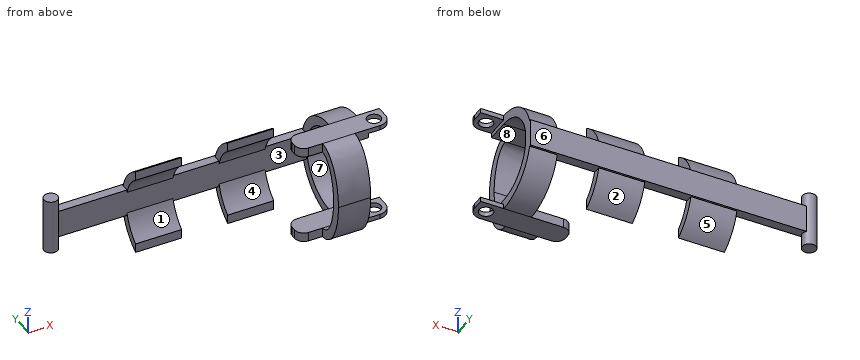
```python
from build123d import *

# Parameters (mm, degrees)
SKETCH1_W                = 2
SKETCH1_H                = 5
BOSS_EXTRUDE1_DEPTH      = 15
BOSS_EXTRUDE1_2_DEPTH    = 15
SKETCH2_W                = 1
SKETCH2_H                = 5
BOSS_EXTRUDE2_DEPTH      = 5
CUT_EXTRUDE1_DEPTH       = 30.107559156
CUT_EXTRUDE1_DEPTH_BACK  = 30.107559156
SKETCH3_R                = 1.5
SWEEP1_START             = 9
SWEEP1_DEPTH             = 6
BOSS_EXTRUDE3_DEPTH      = 12
CUT_EXTRUDE2_DEPTH       = 5
FILLET1_R                = 2
BOSS_EXTRUDE6_START      = -6
SKETCH7_W                = 6
SKETCH7_H                = 2
BOSS_EXTRUDE6_DEPTH      = 61
BOSS_EXTRUDE7_DEPTH      = 3
BOSS_EXTRUDE7_DEPTH_BACK = 9
SKETCH8_R                = 1.5
FILLET2_R                = 2.5
BOSS_EXTRUDE10_DEPTH     = 10
LPATTERN1_COUNT          = 2
LPATTERN1_PITCH          = 20


# Read off the part's stored shape, not the designer's step: Sweep1
with BuildPart() as part:
    # Sketch1 → Boss-Extrude1 (new body)
    with BuildSketch(Plane(origin=(0, 0, 0), x_dir=(0, 0, -1), z_dir=(1, 0, 0))):
        with Locations((-10, 0)):
            Rectangle(SKETCH1_W, SKETCH1_H)
    extrude(amount=BOSS_EXTRUDE1_DEPTH)



with BuildPart() as body_2:
    # Sketch1 → Boss-Extrude1 2 (new body)
    with BuildSketch(Plane(origin=(0, 0, 0), x_dir=(0, 0, -1), z_dir=(1, 0, 0))):
        with Locations((10, 0)):
            Rectangle(SKETCH1_W, SKETCH1_H)
    extrude(amount=BOSS_EXTRUDE1_2_DEPTH)


with BuildPart() as part_1:
    add(part.part)

    add(body_2.part)  # Boss-Extrude2 merges body 2
    # Sketch2 → Boss-Extrude2 (add)
    with BuildSketch(Plane(origin=(15, 0, 0), x_dir=(0, 0, -1), z_dir=(1, 0, 0))):
        with Locations((10.5, 0)):
            Rectangle(SKETCH2_W, SKETCH2_H)
        with Locations((-10.5, 0)):
            Rectangle(SKETCH2_W, SKETCH2_H)
    extrude(amount=BOSS_EXTRUDE2_DEPTH)

    # Sketch3 → Cut-Extrude1 (cut, two sides: drawn at the far end of the back side and taken through both)
    with BuildSketch(Plane.XY.offset(-10).offset(-CUT_EXTRUDE1_DEPTH_BACK)):
        with Locations((17.5, 0)):
            Circle(SKETCH3_R)
    extrude(amount=CUT_EXTRUDE1_DEPTH + CUT_EXTRUDE1_DEPTH_BACK, mode=Mode.SUBTRACT)

    # Sweep1 outline → Sweep1 (add)
    with BuildSketch(Plane.YZ.offset(SWEEP1_START)):
        with BuildLine():
            ThreePointArc((2.5, -11), (13.5, 0), (2.5, 11))
            Line((2.5, 11), (2.5, 9))
            ThreePointArc((2.5, 9), (11.5, 0), (2.5, -9))
            Line((2.5, -9), (2.5, -11))
        make_face()
    extrude(amount=SWEEP1_DEPTH)

    # Sketch5 → Boss-Extrude3 (add)
    with BuildSketch(Plane(origin=(0, 0, 0), x_dir=(0, 0, -1), z_dir=(1, 0, 0))):
        with BuildLine():
            Line((-9, -2.5), (-11, -2.5))
            add(Edge.make_bspline(
                [(-11, -2.5), (-11, -8.980170496), (0, -8.980170496)],
                knots=[3.141592654, 3.141592654, 3.141592654, 4.71238898, 4.71238898, 4.71238898], degree=2, weights=[1, 0.707106781, 1]))
            Line((0, -8.980170496), (0, -7.009343108))
            add(Edge.make_bspline(
                [(-9, -2.5), (-9, -7.009343108), (0, -7.009343108)],
                knots=[3.141592654, 3.141592654, 3.141592654, 4.71238898, 4.71238898, 4.71238898], degree=2, weights=[1, 0.707106781, 1]))
        make_face()
    boss_extrude3 = extrude(amount=BOSS_EXTRUDE3_DEPTH)

    # Sketch6 → Cut-Extrude2 (cut)
    with BuildSketch(Plane.ZY):
        with BuildLine():
            Line((11, -2.5), (9, -2.5))
            add(Edge.make_bspline(
                [(0, -7.009343108), (9, -7.009343108), (9, -2.5)],
                knots=[4.71238898, 4.71238898, 4.71238898, 6.283185307, 6.283185307, 6.283185307], degree=2, weights=[1, 0.707106781, 1]))
            Line((0, -7.009343108), (0, -8.980170496))
            add(Edge.make_bspline(
                [(0, -8.980170496), (11, -8.980170496), (11, -2.5)],
                knots=[4.71238898, 4.71238898, 4.71238898, 6.283185307, 6.283185307, 6.283185307], degree=2, weights=[1, 0.707106781, 1]))
        make_face()
    cut_extrude2 = extrude(amount=-CUT_EXTRUDE2_DEPTH, mode=Mode.SUBTRACT)

    # Mirror2: Boss-Extrude3, Cut-Extrude2 across plane
    add(boss_extrude3.mirror(Plane(origin=(12, -8.980170496, 0), x_dir=(1, 0, 0), z_dir=(0, 0, 1))))
    add(cut_extrude2.mirror(Plane(origin=(12, -8.980170496, 0), x_dir=(1, 0, 0), z_dir=(0, 0, 1))), mode=Mode.SUBTRACT)

    # Fillet1
    fillet1_edges = [part_1.edges().sort_by_distance(p)[0] for p in [
        (0, -2.5, -10),
        (0, 2.5, -10),
        (0, 2.5, 10),
        (0, -2.5, 10),
    ]]
    fillet(fillet1_edges, radius=FILLET1_R)

    # Sketch7 → Boss-Extrude6 (add)
    with BuildSketch(Plane.ZY.offset(-9).offset(BOSS_EXTRUDE6_START)):
        with Locations((0, 12.5)):
            Rectangle(SKETCH7_W, SKETCH7_H)
    extrude(amount=BOSS_EXTRUDE6_DEPTH)

    # Sketch8 → Boss-Extrude7 (add, two sides: drawn at the far end of the back side and taken through both)
    with BuildSketch(Plane.XY.offset(3).offset(-BOSS_EXTRUDE7_DEPTH_BACK)):
        with Locations((-46, 12.5)):
            Circle(SKETCH8_R)
    extrude(amount=BOSS_EXTRUDE7_DEPTH + BOSS_EXTRUDE7_DEPTH_BACK)

    # Fillet2
    fillet2_edges = [part_1.edges().sort_by_distance(p)[0] for p in [
        (20, -2.5, -10.5),
        (20, -2.5, 10.5),
    ]]
    fillet(fillet2_edges, radius=FILLET2_R)

    # 3DSketch3 → Boss-Extrude10 (add)
    with BuildSketch(Plane(origin=(-10, 7.995255445, 9.529017137), x_dir=(0, 0, -1), z_dir=(1, 0, 0))):
        with BuildLine():
            Line((0, 0), (2, 0))
            ThreePointArc((2, 0), (9.529017137, 3.825899604), (17.058034273, 0))
            Line((17.058034273, 0), (19.058034273, 0))
            ThreePointArc((19.058034273, 0), (15.031388903, 4.029654263), (9.529017137, 5.504744555))
            ThreePointArc((9.529017137, 5.504744555), (4.026645371, 4.029654263), (0, 0))
        make_face()
    boss_extrude10 = extrude(amount=BOSS_EXTRUDE10_DEPTH)

    # LPattern1: Boss-Extrude10 ×2
    with Locations(*[(-i * LPATTERN1_PITCH, 0, 0) for i in range(1, LPATTERN1_COUNT)]):
        add(boss_extrude10)


solid = part_1.part
```
Here's how the part is built. I have some questions about the finished solid (model axes, mm). Face numbers are marked on the shaded views. A direction names the side the tool comes from. Round coordinates to 2 decimals unless told otherwise and drop trailing zeros. Order: outer loops, then holes, each group sorted by start corner. A loop starts at its lowest first (then second) coordinate and runs counter-clockwise, first axis right, second up. Notation, with made-up numbers: M -37.5,70.25 L -26.5,70.25 A24 ccw -26.5,95.25 Z; hole C 87,55.5 d6. An arc over 180 degrees is marked long. Use CSV: the item, a comma, the result in double quotes.
1) I want a section at A-A (x = 4). List the corners of the cut face in (y, z) for me.
Taken from the geometry:
outline,"M -2.5,-11 L 2.5,-11 L 2.5,-9 L -2.5,-9 Z; M -2.5,9 L 2.5,9 L 2.5,11 L -2.5,11 Z; M 11.5,-3 L 13.5,-3 L 13.5,3 L 11.5,3 Z"
2) I need wall thicknesses on line 1 along Y through (x, z) = (17.5, 10.4); line 2 along X through (y, z) = (0, 10.75); line 3 along Y through (x, z) = (11, 0). Which ranges of each line are inside material? Lowest first, please. Write a range as [from, to].
Taken from the geometry:
line 1,"[-2.5, -1.5], [1.5, 2.5]"
line 2,"[0, 16], [19, 20]"
line 3,"[-8.98, -7.01], [11.5, 13.5]"
3) I'm going to push flat-ended pins straight in: P1, Ø3, axis at x = -8, z = 6.5, coming from the +Y side; P2, Ø2.5, axis at x = -46.5, y = 12.5, coming from the +Z side; P3, Ø2, axis at x = -16, y = 12, coming from the +Z side. Where does each tip first touch, or does it pass through?
Taken from the geometry:
P1,"y = 12.3"
P2,"z = 6"
P3,"z = 3"
4) If we mould it in two halves opening along X, with no side actions, what happens to the marked faces 1, 2 and 3? For each: pulls with the +X half, pulls with the -X half, needs draft (parallel to the pull), parting line crosses it, or undercut.
Taken from the geometry:
face 1,"undercut"
face 2,"needs draft"
face 3,"undercut"
5) On a 3-axis mill with a long thin cutter (end or side, diameter ignored), from which of +Z, -Z, +X, -X, +Y, -Y can I reach the whole of each face in a straight line? I mean the marked faces 4, 5, 6, 7 and 8. Say none if no direction works.
Taken from the geometry:
face 4,"-Y"
face 5,"-Z, +X, +Y"
face 6,"+Z, -Z, +X, +Y"
face 7,"+X"
face 8,"+X, -X"
6) I want a section at D-D (x = -46). List the corners of the cut face in (y, z) for me, then the cut area to 3 significant figures.
Taken from the geometry:
outline,"M 11,-6 L 14,-6 L 14,6 L 11,6 Z"
area,"36.0 mm^2"
7) I want a section at B-B (y = 3.25). List the corners of the cut face in (x, z) for me.
Taken from the geometry:
outline,"M 9,-10.97 L 15,-10.97 L 15,-8.97 L 9,-8.97 Z; M 9,8.97 L 15,8.97 L 15,10.97 L 9,10.97 Z"
8) I want a section at C-C (z = 4.5). Count the separate pieces of the cut face and the enclosed holes in it, then the cut area to 3 significant figures.
Taken from the geometry:
separate pieces,"5"
enclosed holes,"0"
area,"72.1 mm^2"
